The model under review builds one solid part; all positions refer to its coordinate system, in mm. A direction names the side the tool comes from. Round coordinates to 2 decimals unless told otherwise and drop trailing zeros. Write each loop counter-clockwise with the first axis right and the second up, starting at its lowest first coordinate (ties: lowest second). Pieces come first, ordered by that corner, then holes. Notation, with made-up numbers: (32.25, 64) -> (89.25, 64) arc R22 ccw to (89.25, 76) -> close; hole circle Ø8 at (55.5, -1.75). An arc over 180 degrees is marked (long way). Answer as a JSON object with one key per item and string values. Group by question number.
1) Insertion check: pin 1 Ø1.2 at (x, y) = (55.5, 31) entering from +Z; pin 2 Ø12 at (x, y) = (40.5, 29.5) entering from +Z; pin 3 Ø1.9 at (x, y) = (56, 14) entering from +Z. Each pin has a flat end and moves straight along its axis. Give the tip position at first contact, or say it passes through.
2) Machinability: for faces 4 (the cylindrical face through (0.57, 37.9, 26)), 5 (the cylindrical face through (30.322, 42.938, 6.565)), 6 (the cylindrical face through (30.322, 2.091, 6.587)), which of the approach directions +Z, -Z, +X, -X, +Y, -Y give a long, thin tool a straight path to every point of the face, cutting with its end or side? Answer none if there is none.
3) We need section B-B, the plane x = 54.5. Write out the cut boundary in (y, z), then the cut area to 3 significant figures.
4) To check wall thickness, follow probe 1 along X at (y, z) = (24.5, 20); probe 2 along Z at (x, y) = (16.5, 38); probe 3 along Z at (x, y) = (54, 22). State the ranges of each line that lie inside material, in increasing order. Write a range as [from, to].
5) We need section A-A, the plane x = 21.5. Write out the cut boundary in (y, z), then the cut area to 3 significant figures.
6) Mouldability with a two-part tool opening along X and no side actions: class faces 1 (the flat face through (53, 22, 25)), 2 (the cylindrical face through (4.535, 22.675, 56.464)), 3 (the cylindrical face through (0.6, 22.78, 0.57)) as pulls with the +X half, pulls with the -X half, needs draft (parallel to the pull), parting line crosses it, or undercut.
Autodesk Inventor part; units mm, degrees
ref_plane "YZ Plane" through (0, 0, 0) normal (1, 0, 0) x (0, 1, 0)
ref_plane "XZ Plane" through (0, 0, 0) normal (0, 1, 0) x (-1, 0, 0)
ref_plane "XY Plane" through (0, 0, 0) normal (0, 0, 1) x (1, 0, 0)
sketch "Sketch1" plane through (0, 0, 0) normal (0, 0, 1) x (1, 0, 0)
  point P0 (0, 0)
sketch "Sketch2" plane through (0, 0, 0) normal (0, 0, 1) x (1, 0, 0)
  line L0 (0, 0) -> (60, 0)
  line L1 (60, 0) -> (60, 45)
  line L2 (60, 45) -> (0, 45)
  line L3 (0, 45) -> (0, 0)
  dimension "d0" = 60
  dimension "d1" = 45
extrude "Extrusion1" add sketch "Sketch2" along normal blind 50
sketch "Sketch3" plane through (60, 0, 0) normal (1, 0, 0) x (0, 0, -1)
  line L0 (0, 45) -> (-50, 45)
  line L1 (-50, 0) -> (-50, 45)
  line L2 (0, 0) -> (-50, 0)
  line L3 (0, 45) -> (-50, 32.5336)
  line L4 (0, 45) -> (51.5307, 45) construction
  line L5 (0, 0) -> (-50, 12.4664)
  line L6 (0, 0) -> (51.5307, 0) construction
  dimension "d4" = 166
  dimension "d5" = 166
extrude "Extrusion2" cut sketch "Sketch3" against normal through all
sketch "Sketch4" plane through (60, 0, 0) normal (1, 0, 0) x (0, 0, -1)
  line L0 (-50, 12.4664) -> (-50, 32.5336)
  circle A0 centre (-45.6937, 22.5) radius 10.7721
  point P0 (-50, 32.3739)
  point P1 (-50, 12.6261)
extrude "Extrusion3" add sketch "Sketch4" against normal blind 60 contours A0 L0 picked at (-52.7772, 22.9072)
sketch "Sketch6" plane through (0, 0, 0) normal (0, 0, -1) x (-1, 0, 0)
  line L0 (0, 0) -> (-60, 0)
  line L1 (-60, 45) -> (0, 45)
  line L2 (-7, 0) -> (-53, 0)
  line L3 (-53, 0) -> (-53, 45)
  line L4 (-53, 45) -> (-7, 45)
  line L5 (-7, 45) -> (-7, 0)
  point P0 (-7, 45)
  dimension "d10" = 46
extrude "Extrusion4" cut sketch "Sketch6" against normal through all
sketch "Sketch7" plane through (0, 0, 0) normal (0, 0, -1) x (-1, 0, 0)
  line L0 (-7, 45) -> (-7, 0)
  line L1 (-7, 32.5336) -> (-7, 45)
  line L2 (-53, 0) -> (-60, 0)
  line L3 (-7, 45) -> (-53, 45)
  line L4 (-53, 45) -> (-53, 0)
  line L5 (-53, 0) -> (-7, 0)
  line L6 (-7, 0) -> (-7, 45)
  point P0 (-7, 0)
extrude "Extrusion5" add sketch "Sketch7" against normal blind 7
sketch "Sketch8" plane through (60, 0, 0) normal (1, 0, 0) x (0, 0, -1)
  line L0 (0, 45) -> (-50, 32.5336)
  line L1 (-50, 32.3739) -> (-50, 32.5336)
  arc A0 (-50, 32.3739) -> (-50, 12.6261) centre (-45.6937, 22.5) ccw
  line L2 (-50, 12.4664) -> (-50, 12.6261)
  line L3 (-50, 12.4664) -> (0, 0)
  line L4 (0, 0) -> (0, 45)
sketch "Sketch9" plane through (53, 43.2547, 7) normal (1, 0, 0) x (0, 0, -1)
  line L0 (7, 1.7453) -> (0, 0)
  line L1 (7, 1.7453) -> (0, 1.7453)
  line L2 (0, 0) -> (0, 1.7453)
  line L3 (7, -43.2547) -> (7, 1.7453)
  line L4 (0, 0) -> (7, 1.7453)
  line L5 (7, 1.7453) -> (0, 1.7453)
extrude "Extrusion6" cut sketch "Sketch9" against normal through all
sketch "Sketch10" plane through (53, 0, 7) normal (1, 0, 0) x (0, 0, -1)
  line L0 (0, 1.7453) -> (7, 0)
  line L1 (0, 0) -> (0, 1.7453)
  line L2 (7, 0) -> (0, 0)
  line L3 (-43, 12.4664) -> (7, 0)
  line L4 (0, 43.2547) -> (0, 1.7453)
  line L5 (7, 0) -> (0, 1.7453)
  line L6 (0, 1.7453) -> (0, 0)
extrude "Extrusion7" cut sketch "Sketch10" against normal through all
fillet "Fillet1" radius 2 12 edges at (60, 6.2332, 25) (60, 22.5, 56.4658) (60, 38.7668, 25) (60, 22.5, 0) (30, 0, 0) (30, 45, 0) (0, 22.5, 0) (0, 6.2332, 25) (0, 22.5, 56.4658) (0, 38.7668, 25) (30, 43.2547, 7) (30, 1.7453, 7)
properties part number "schouder(s)"
Here are the results:
{
 "1": {"pin 1": "stops at z = 53.02", "pin 2": "stops at z = 7", "pin 3": "stops at z = 53.38"},
 "2": {"face 4": "+Z, -X, +Y", "face 5": "+Z, +Y", "face 6": "+Z, -Y"},
 "3": {"outline": "(0.62, 2.48) arc R2 ccw to (2.56, 0) -> (42.44, 0) arc R2 ccw to (44.38, 2.48) -> (32.53, 50) -> (32.37, 50) arc R10.77 ccw to (12.63, 50) -> (12.47, 50) -> close", "area": "1,720 mm^2"},
 "4": {"probe 1": "x = [0, 7], [53, 60]", "probe 2": "z = [0, 7]", "probe 3": "z = [0, 56.45]"},
 "5": {"outline": "(0.62, 2.48) arc R2 ccw to (2.56, 0) -> (42.44, 0) arc R2 ccw to (44.38, 2.48) -> (43.63, 5.48) arc R2 ccw to (41.69, 7) -> (3.31, 7) arc R2 ccw to (1.37, 5.48) -> close", "area": "299 mm^2"},
 "6": {"face 1": "undercut", "face 2": "needs draft", "face 3": "pulls with the -X half"}
}
